Source: CAD feature listing. Evaluate the final solid. Frame: model axes, mm. Give positions to 0.01 mm unless a question says otherwise; leave off trailing zeros. Write each loop counter-clockwise with the first axis right and the second up, starting at its lowest first coordinate (ties: lowest second). Pieces come first, ordered by that corner, then holes. Notation, with made-up numbers: (5.25, 60) -> (36.25, 60) arc R29 cw to (36.25, 89) -> close; hole circle Ø9 at (60, -36). An arc over 180 degrees is marked (long way). Write item = value, one per line.
from build123d import *

# Parameters (mm, degrees)
F1_DEPTH = 20
F2_DEPTH = 21
F3_DEPTH = 18
F4_DEPTH = 10
F10_R    = 1
F6_SIZE  = 0.99999
F7_SIZE  = 1
F8_SIZE  = 1
F9_SIZE  = 2.5


# Not quite as in the source:
# - a fillet or chamfer that OpenCascade refuses, or shapes differently, is made with other operations: its cross-section is extruded or revolved along the edge and cut away or added
# - a fillet or chamfer is up to 0.001 mm smaller than in the source, because OpenCascade refuses the exact size


with BuildPart() as f1:
    # F0 (on Top) → F1 (new body)
    with BuildSketch(Plane.XY):
        with BuildLine():
            ThreePointArc((3, 0), (2.9840537841, 0.308906157), (2.9363846575, 0.6145283911))
            Line((2.9363846575, 0.6145283911), (2.9363846575, -0.6145283911))
            ThreePointArc((2.9363846575, -0.6145283911), (2.9840537841, -0.308906157), (3, 0))
        make_face()
        with BuildLine():
            Line((5.5474227354, 0.6145283911), (7.4747812581, 0.6145283911))
            ThreePointArc((7.4747812581, 0.6145283911), (-7.5, 0), (7.4747812581, -0.6145283911))
            Line((7.4747812581, -0.6145283911), (5.5474227354, -0.6145283911))
            ThreePointArc((5.5474227354, -0.6145283911), (-5.5813568376, 0), (5.5474227354, 0.6145283911))
        make_face()
        with BuildLine():
            Line((2.9363846575, 0.6145283911), (5.5474227354, 0.6145283911))
            ThreePointArc((5.5474227354, 0.6145283911), (-5.5813568376, 0), (5.5474227354, -0.6145283911))
            Line((5.5474227354, -0.6145283911), (2.9363846575, -0.6145283911))
            ThreePointArc((2.9363846575, -0.6145283911), (-3, 0), (2.9363846575, 0.6145283911))
        make_face()
        with BuildLine():
            Line((2.9363846575, -0.6145283911), (2.9363846575, 0.6145283911))
            ThreePointArc((2.9363846575, 0.6145283911), (-3, 0), (2.9363846575, -0.6145283911))
        make_face()
        with BuildLine():
            ThreePointArc((7.4747812581, -0.6145283911), (7.4936926624, -0.3075228156), (7.5, 0))
            ThreePointArc((7.5, 0), (7.4936926624, 0.3075228156), (7.4747812581, 0.6145283911))
            Line((7.4747812581, 0.6145283911), (5.5474227354, 0.6145283911))
            ThreePointArc((5.5474227354, 0.6145283911), (5.5728668548, 0.3077322971), (5.5813568376, 0))
            ThreePointArc((5.5813568376, 0), (5.5728668548, -0.3077322971), (5.5474227354, -0.6145283911))
            Line((5.5474227354, -0.6145283911), (7.4747812581, -0.6145283911))
        make_face()
        with BuildLine():
            ThreePointArc((5.5813568376, 0), (5.5728668548, 0.3077322971), (5.5474227354, 0.6145283911))
            Line((5.5474227354, 0.6145283911), (2.9363846575, 0.6145283911))
            ThreePointArc((2.9363846575, 0.6145283911), (2.9840537841, 0.308906157), (3, 0))
            ThreePointArc((3, 0), (2.9840537841, -0.308906157), (2.9363846575, -0.6145283911))
            Line((2.9363846575, -0.6145283911), (5.5474227354, -0.6145283911))
            ThreePointArc((5.5474227354, -0.6145283911), (5.5728668548, -0.3077322971), (5.5813568376, 0))
        make_face()
    extrude(amount=F1_DEPTH)

    # F0 (on Top) → F2 (join)
    with BuildSketch(Plane.XY):
        with BuildLine():
            ThreePointArc((7.4747812581, 0.6145283911), (7.4936926624, 0.3075228156), (7.5, 0))
            ThreePointArc((7.5, 0), (7.4936926624, -0.3075228156), (7.4747812581, -0.6145283911))
            Line((7.4747812581, -0.6145283911), (8.0371221235, -0.6145283911))
            Line((8.0371221235, -0.6145283911), (8.0371221235, 0.6145283911))
            Line((8.0371221235, 0.6145283911), (7.4747812581, 0.6145283911))
        make_face()
        with BuildLine():
            ThreePointArc((7.4747812581, -0.6145283911), (7.4936926624, -0.3075228156), (7.5, 0))
            ThreePointArc((7.5, 0), (7.4936926624, 0.3075228156), (7.4747812581, 0.6145283911))
            Line((7.4747812581, 0.6145283911), (5.5474227354, 0.6145283911))
            ThreePointArc((5.5474227354, 0.6145283911), (5.5728668548, 0.3077322971), (5.5813568376, 0))
            ThreePointArc((5.5813568376, 0), (5.5728668548, -0.3077322971), (5.5474227354, -0.6145283911))
            Line((5.5474227354, -0.6145283911), (7.4747812581, -0.6145283911))
        make_face()
        with BuildLine():
            ThreePointArc((5.5813568376, 0), (5.5728668548, 0.3077322971), (5.5474227354, 0.6145283911))
            Line((5.5474227354, 0.6145283911), (2.9363846575, 0.6145283911))
            ThreePointArc((2.9363846575, 0.6145283911), (2.9840537841, 0.308906157), (3, 0))
            ThreePointArc((3, 0), (2.9840537841, -0.308906157), (2.9363846575, -0.6145283911))
            Line((2.9363846575, -0.6145283911), (5.5474227354, -0.6145283911))
            ThreePointArc((5.5474227354, -0.6145283911), (5.5728668548, -0.3077322971), (5.5813568376, 0))
        make_face()
    extrude(amount=F2_DEPTH)

    # F0 (on Top) → F3 (cut)
    with BuildSketch(Plane.XY):
        with BuildLine():
            Line((2.9363846575, -0.6145283911), (2.9363846575, 0.6145283911))
            ThreePointArc((2.9363846575, 0.6145283911), (-3, 0), (2.9363846575, -0.6145283911))
        make_face()
        with BuildLine():
            ThreePointArc((3, 0), (2.9840537841, 0.308906157), (2.9363846575, 0.6145283911))
            Line((2.9363846575, 0.6145283911), (2.9363846575, -0.6145283911))
            ThreePointArc((2.9363846575, -0.6145283911), (2.9840537841, -0.308906157), (3, 0))
        make_face()
    extrude(amount=F3_DEPTH, mode=Mode.SUBTRACT)

    # F0 (on Top) → F4 (cut)
    with BuildSketch(Plane.XY):
        with BuildLine():
            Line((2.9363846575, 0.6145283911), (5.5474227354, 0.6145283911))
            ThreePointArc((5.5474227354, 0.6145283911), (-5.5813568376, 0), (5.5474227354, -0.6145283911))
            Line((5.5474227354, -0.6145283911), (2.9363846575, -0.6145283911))
            ThreePointArc((2.9363846575, -0.6145283911), (-3, 0), (2.9363846575, 0.6145283911))
        make_face()
        with BuildLine():
            ThreePointArc((5.5813568376, 0), (5.5728668548, 0.3077322971), (5.5474227354, 0.6145283911))
            Line((5.5474227354, 0.6145283911), (2.9363846575, 0.6145283911))
            ThreePointArc((2.9363846575, 0.6145283911), (2.9840537841, 0.308906157), (3, 0))
            ThreePointArc((3, 0), (2.9840537841, -0.308906157), (2.9363846575, -0.6145283911))
            Line((2.9363846575, -0.6145283911), (5.5474227354, -0.6145283911))
            ThreePointArc((5.5474227354, -0.6145283911), (5.5728668548, -0.3077322971), (5.5813568376, 0))
        make_face()
    extrude(amount=F4_DEPTH, mode=Mode.SUBTRACT)

    # F10
    f10_edges = [f1.edges().sort_by_distance(p)[0] for p in [
        (-7.5, 0, 20),
        (8.037122, 0, 21),
    ]]
    fillet(f10_edges, radius=F10_R)

    # F5: chamfer of 3 on 1 edges, made by hand

    # F5_s1 → F5_t2 (revolve)
    with BuildSketch(Plane(origin=(0, 0, 0), x_dir=(0, 0, 1), z_dir=(-0.204842797, -0.9787948858, 0))):
        Polygon((15, -3), (18, 0), (18, -3), align=None)
    revolve(axis=Axis((0, 0, 18), (0, 0, 1)))

    # F6 (size 1 in the source; OpenCascade refuses exactly that, so slightly less here)
    f6_edges = [f1.edges().sort_by_distance(p)[0] for p in [
        (3, 0, 21),
    ]]
    chamfer(f6_edges, length=F6_SIZE)

    # F7
    f7_edges = [f1.edges().sort_by_distance(p)[0] for p in [
        (-7.5, 0, 0),
    ]]
    chamfer(f7_edges, length=F7_SIZE)

    # F8
    f8_edges = [f1.edges().sort_by_distance(p)[0] for p in [
        (8.037122, 0, 0),
    ]]
    chamfer(f8_edges, length=F8_SIZE)

    # F9
    f9_edges = [f1.edges().sort_by_distance(p)[0] for p in [
        (-5.547423, 0.614528, 10),
    ]]
    chamfer(f9_edges, length=F9_SIZE)


solid = f1.part
(1) Pull-direction query (X, two-part tool) for faces 1 (the face through (8.037, 0, 10)), 2 (the face through (-3, 5, 0)), 3 (the face through (0, 1, 17)); classes: pulls with the +X half, pulls with the -X half, needs draft (parallel to the pull), parting line crosses it, or undercut.
Values follow:
face_1 = pulls with the +X half
face_2 = needs draft
face_3 = undercut
(2) Section query B-B (z = 8.75). Return loops of the section in (x, y), plus the area to 3 significant figures.
Values follow:
outline = (7.47, -0.61) -> (8.04, -0.61) -> (8.04, 0.61) -> (7.47, 0.61) arc R7.5 ccw (long way) to start; hole circle Ø8.66 at (0, 0)
area = 118 mm2
(3) First-contact query: pin 1 (4 mm diameter, centred on x = 6.5, z = 14, fed in from +Y); pin 2 (5 mm diameter, centred on x = 0, y = 0, fed in from -Z); pin 3 (2 mm diameter, centred on y = -6, z = 16, fed in from +X); pin 4 (6 mm diameter, centred on x = -3, z = 3, fed in from -Y). Flat tips, straight axial feed; report the tip coordinate or a pass-through.
Values follow:
pin_1 = 6
pin_2 = 15.5
pin_3 = 5.59
pin_4 = -7.5
(4) Material intervals for line 1 (Y direction, x = 0, z = 5.75); line 2 (X direction, y = 0, z = 5.5); line 3 (Y direction, x = 0, z = 13.2), sorted ascending.
Values follow:
line_1 = -7.5 to -5.58, 5.58 to 7.5
line_2 = -7.5 to -5.58, 5.58 to 8.04
line_3 = -7.5 to -3, 3 to 7.5
(5) Section query A-A (z = 5.5). Return loops of the section in (x, y), plus the area to 3 significant figures.
Values follow:
outline = (7.47, -0.61) -> (8.04, -0.61) -> (8.04, 0.61) -> (7.47, 0.61) arc R7.5 ccw (long way) to start; hole circle Ø11.16 at (0, 0)
area = 79.5 mm2
